from build123d import *

# Parameters (mm, degrees)
F0_W      = 110
F0_H      = 51
F0_W_2    = 105
F0_H_2    = 46
F1_DEPTH  = 75
F3_DEPTH  = 16
F5_W      = 1
F5_H      = 3
F6_DEPTH  = 8
F8_W      = 2.5
F8_H      = 3
F9_DEPTH  = 16
F12_DEPTH = 5
F15_D     = 2
F15_DEPTH = 12
F15_TIP   = 0.600860619
F16_W     = 28
F16_H     = 47
F17_DEPTH = 12.5
F19_W     = 105
F19_H     = 46
F20_DEPTH = 1.5
F22_D     = 12
F22_DEPTH = 12
F22_TIP   = 3.6051637142
F14_R     = 1.15
F14_R_2   = 0.85
F23_DEPTH = 0.5
F25_D     = 2
F25_DEPTH = 12
F25_TIP   = 0.600860619
F24_R     = 1.15
F24_R_2   = 0.85
F26_DEPTH = 0.5


# Not quite as in the source:
# - a feature names something its author has since deleted; it is built from what else it names


with BuildPart() as f1:
    # F0 (on Top) → F1 (new body)
    with BuildSketch(Plane.XY):
        with Locations((14.1399928927, -8.9340824737)):
            Rectangle(F0_W, F0_H)
        with Locations((14.1399928927, -8.9340824737)):
            Rectangle(F0_W_2, F0_H_2, mode=Mode.SUBTRACT)
    extrude(amount=F1_DEPTH)


with BuildPart() as f3:
    # F2 (on face) → F3 (new body)
    with BuildSketch(Plane.XY):
        Polygon((-39.3600071073, -34.4340824737), (-39.3600071073, 15.0659175263), (69.1399928927, 15.0659175263), (69.1399928927, 16.5659175263), (-40.8600071073, 16.5659175263), (-40.8600071073, -34.4340824737), align=None)
    extrude(amount=F3_DEPTH)


with BuildPart() as f1_1:
    add(f1.part)

    # F4: cut F3
    add(f3.part, mode=Mode.SUBTRACT)


with BuildPart() as f6:
    # F5 (on face) → F6 (new body)
    with BuildSketch(Plane.XY):
        with Locations((-38.8600071073, 9.5659175263)):
            Rectangle(F5_W, F5_H)
    extrude(amount=F6_DEPTH)


with BuildPart() as f1_2:
    add(f1_1.part)

    # F7: cut F6
    add(f6.part, mode=Mode.SUBTRACT)


with BuildPart() as f9:
    # F8 (on face) → F9 (new body)
    with BuildSketch(Plane.XY):
        with Locations((67.8899928927, 9.5659175263)):
            Rectangle(F8_W, F8_H)
    extrude(amount=F9_DEPTH)


with BuildPart() as f1_3:
    add(f1_2.part)

    # F10: cut F9
    add(f9.part, mode=Mode.SUBTRACT)


with BuildPart() as f12:
    # F11 (on face) → F12 (new body, symmetric)
    with BuildSketch(Plane.XZ.offset(-14.0659175263)):
        with BuildLine():
            Line((62.6399928927, 0), (62.6399928927, 11))
            ThreePointArc((62.6399928927, 11), (60.1399928927, 8.5), (57.6399928927, 11))
            Line((57.6399928927, 11), (57.6399928927, 0))
            Line((57.6399928927, 0), (62.6399928927, 0))
        make_face()
        with BuildLine():
            ThreePointArc((57.6399928927, 11), (60.1399928927, 8.5), (62.6399928927, 11))
            ThreePointArc((62.6399928927, 11), (60.1399928927, 13.5), (57.6399928927, 11))
        make_face()
    extrude(amount=F12_DEPTH, both=True)


with BuildPart() as f1_4:
    add(f1_3.part)

    # F13: cut F12
    add(f12.part, mode=Mode.SUBTRACT)

    # F15
    with Locations(Plane(origin=(-39.3600071073, 0, 0), x_dir=(0, -1, 0), z_dir=(-1, 0, 0))):
        with Locations((27.9340824737, 9.5), (17.9340824737, 9.5)):
            Hole(F15_D / 2, depth=F15_DEPTH)
            with Locations((0, 0, -(F15_DEPTH + F15_TIP / 2))):  # 118° drill point
                Cone(0, F15_D / 2, F15_TIP, mode=Mode.SUBTRACT)


with BuildPart() as f17:
    # F16 (on face) → F17 (new body, symmetric)
    with BuildSketch(Plane(origin=(-40.8600071073, 0, 0), x_dir=(0, -1, 0), z_dir=(-1, 0, 0))):
        with Locations((8.9340824737, 45.5)):
            Rectangle(F16_W, F16_H)
    extrude(amount=F17_DEPTH, both=True)


with BuildPart() as f1_5:
    add(f1_4.part)

    # F18: cut F17
    add(f17.part, mode=Mode.SUBTRACT)

    # F19 (on face) → F20 (join)
    with BuildSketch(Plane.XY.offset(75)):
        with Locations((14.1399928927, -8.9340824737)):
            Rectangle(F19_W, F19_H)
    extrude(amount=-F20_DEPTH)

    # F22
    with Locations(Plane.XZ.offset(34.4340824737)):
        with Locations((59.1399928927, 15)):
            Hole(F22_D / 2, depth=F22_DEPTH)
            with Locations((0, 0, -(F22_DEPTH + F22_TIP / 2))):  # 118° drill point
                Cone(0, F22_D / 2, F22_TIP, mode=Mode.SUBTRACT)

    # F14 (on face) → F23 (join)
    with BuildSketch(Plane(origin=(-39.3600071073, 0, 0), x_dir=(0, -1, 0), z_dir=(-1, 0, 0))):
        with Locations((27.9340824737, 9.5)):
            Circle(F14_R)
        with Locations((27.9340824737, 9.5)):
            Circle(F14_R_2, mode=Mode.SUBTRACT)
        with Locations((17.9340824737, 9.5)):
            Circle(F14_R)
        with Locations((17.9340824737, 9.5)):
            Circle(F14_R_2, mode=Mode.SUBTRACT)
    extrude(amount=F23_DEPTH)

    # F25
    with Locations(Plane(origin=(0, 15.0659175263, 0), x_dir=(-1, 0, 0), z_dir=(0, 1, 0))):
        with Locations((35.8600071073, 11)):
            Hole(F25_D / 2, depth=F25_DEPTH)
            with Locations((0, 0, -(F25_DEPTH + F25_TIP / 2))):  # 118° drill point
                Cone(0, F25_D / 2, F25_TIP, mode=Mode.SUBTRACT)

    # F24 (on face) → F26 (join)
    with BuildSketch(Plane(origin=(0, 15.0659175263, 0), x_dir=(-1, 0, 0), z_dir=(0, 1, 0))):
        with Locations((35.8600071073, 11)):
            Circle(F24_R)
        with Locations((35.8600071073, 11)):
            Circle(F24_R_2, mode=Mode.SUBTRACT)
    extrude(amount=F26_DEPTH)


solid = f1_5.part
Work out the finished part from the listing and answer in its coordinate system (mm). A direction names the side the tool comes from. Give positions to 0.01 mm unless a question says otherwise; leave off trailing zeros. Loops run counter-clockwise (first coordinate to the right, second up) from the corner with the lowest first, then second, coordinate; pieces in that order, holes last. Notation, with made-up numbers: (60, 83) - (75, 83) arc R16 ccw to (75, 104) - close; hole circle Ø4 at (59, 83). An arc over 180 degrees is marked (long way). Answer in a Markdown table with one row per item.
(1) Section B-B (x = 56) is taken. Give the vertices of the cut face in (y, z).
Results list:
| item | result |
|---|---|
| outline | (-34.43, 0) - (-31.93, 0) - (-31.93, 9.89) - (-34.43, 9.89) - close; (-34.43, 20.11) - (-31.93, 20.11) - (-31.93, 73.5) - (14.07, 73.5) - (14.07, 0) - (15.07, 0) - (15.07, 16) - (16.57, 16) - (16.57, 75) - (-34.43, 75) - close |
(2) Section D-D (x = 7.5) is taken. Give the vertices of the cut face in (y, z), and give its area (3 significant figures).
Results list:
| item | result |
|---|---|
| outline | (-34.43, 0) - (-31.93, 0) - (-31.93, 73.5) - (14.07, 73.5) - (14.07, 0) - (15.07, 0) - (15.07, 16) - (16.57, 16) - (16.57, 75) - (-34.43, 75) - close |
| area | 420 mm² |
(3) For a pull along X with two mould halves and no side action, classify faces 5 (the face through (-38.36, -9, 20)), 6 (the face through (-36.922, 15.312, 10.56)), 7 (the face through (13, 16.566, 45)) as pulls with the +X half, pulls with the -X half, needs draft (parallel to the pull), parting line crosses it, or undercut.
Results list:
| item | result |
|---|---|
| face 5 | undercut |
| face 6 | parting line crosses it |
| face 7 | needs draft |
(4) Section C-C (z = 32) is taken. Give the vertices of the cut face in (x, y), and give its area (3 significant figures).
Results list:
| item | result |
|---|---|
| outline | (-40.86, -34.43) - (69.14, -34.43) - (69.14, 16.57) - (-40.86, 16.57) - (-40.86, 5.07) - (-38.36, 5.07) - (-38.36, 14.07) - (66.64, 14.07) - (66.64, -31.93) - (-38.36, -31.93) - (-38.36, -22.93) - (-40.86, -22.93) - close |
| area | 710 mm² |
(5) Flat-ended cylindrical pins translate along their axes: pin 1 Ø0.7 at (y, z) = (-27.5, 9.5) entering from -X; pin 2 Ø1.1 at (x, y) = (-39, 10) entering from -Z; pin 3 Ø0.8 at (x, z) = (-38.5, 4) entering from +Y. Find the tip coordinate at first contact, or state that the pin passes through.
Results list:
| item | result |
|---|---|
| pin 1 | stops at x = 66.64 |
| pin 2 | stops at z = 8 |
| pin 3 | stops at y = 15.07 |
(6) Consider L1, parallel to X at y = -13.5, z = 7; L2, parallel to Y at x = 44, z = 47; L3, parallel to X at y = 7.5, z = 53. Determine where each line is inside the solid, lowest interval first. Write a range as [from, to].
Results list:
| item | result |
|---|---|
| L1 | x = [-39.36, -38.36], [66.64, 69.14] |
| L2 | y = [-34.43, -31.93], [14.07, 16.57] |
| L3 | x = [-40.86, -38.36], [66.64, 69.14] |
(7) A tool of negligible diameter and unlimited length cuts with its end or side. For faces 1 (the face through (53.6, -33.2, 12.7)), 2 (the face through (13, -9, 75)), 3 (the face through (68, 10, 16)), 4 (the face through (-39.6, -18.5, 8.5)), from which of +Z, -Z, +X, -X, +Y, -Y can it reach the whole face along a straight path? Write none if from no direction.
Results list:
| item | result |
|---|---|
| face 1 | -Y |
| face 2 | +Z, +X, -X, +Y, -Y |
| face 3 | -Z, +X |
| face 4 | -X |
(8) Section A-A (y = -5.5) is taken. Give the vertices of the cut face in (x, z), and give its area (3 significant figures).
Results list:
| item | result |
|---|---|
| outline | (-40.86, 16) - (-39.36, 16) - (-39.36, 0) - (-38.36, 0) - (-38.36, 22) - (-40.86, 22) - close; (-40.86, 69) - (-38.36, 69) - (-38.36, 73.5) - (66.64, 73.5) - (66.64, 0) - (69.14, 0) - (69.14, 75) - (-40.86, 75) - close |
| area | 391 mm² |
